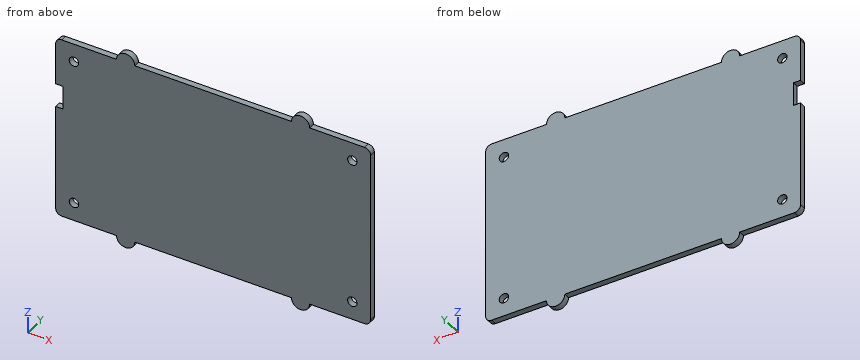
from build123d import *

# Parameters (mm, degrees)
SKETCH_1_R      = 1.55
EXTRUDE_1_DEPTH = 2


with BuildPart() as part:
    # 草图1 → 凸台-拉伸1 (new body)
    with BuildSketch(Plane(origin=(0, 0, 0), x_dir=(1, 0, 0), z_dir=(0, 1, 0))):
        with BuildLine():
            Line((97.46, -4), (97.46, 52.29))
            ThreePointArc((97.46, 52.29), (96.874213562, 53.704213562), (95.46, 54.29))
            Line((95.46, 54.29), (77.46, 54.29))
            ThreePointArc((77.46, 54.29), (74.46, 57.29), (71.46, 54.29))
            Line((71.46, 54.29), (20, 54.29))
            ThreePointArc((20, 54.29), (17, 57.29), (14, 54.29))
            Line((14, 54.29), (-4, 54.29))
            ThreePointArc((-4, 54.29), (-5.414213562, 53.704213562), (-6, 52.29))
            Line((-6, 52.29), (-6, 17.493898271))
            Line((-6, 17.493898271), (-3.6, 17.493898271))
            Line((-3.6, 17.493898271), (-3.6, 9.75))
            Line((-3.6, 9.75), (-6, 9.75))
            Line((-6, 9.75), (-6, -4))
            ThreePointArc((-6, -4), (-5.414213562, -5.414213562), (-4, -6))
            Line((-4, -6), (14, -6))
            ThreePointArc((14, -6), (17, -9), (20, -6))
            Line((20, -6), (71.46, -6))
            ThreePointArc((71.46, -6), (74.46, -9), (77.46, -6))
            Line((77.46, -6), (95.46, -6))
            ThreePointArc((95.46, -6), (96.874213562, -5.414213562), (97.46, -4))
        make_face()
        Circle(SKETCH_1_R, mode=Mode.SUBTRACT)
        with Locations((91.46, 0)):
            Circle(SKETCH_1_R, mode=Mode.SUBTRACT)
        with Locations((0, 48.29)):
            Circle(SKETCH_1_R, mode=Mode.SUBTRACT)
        with Locations((91.46, 48.29)):
            Circle(SKETCH_1_R, mode=Mode.SUBTRACT)
    extrude(amount=EXTRUDE_1_DEPTH)


solid = part.part
Geometry check sheet. Reference: the model listing, model coordinates, mm. Round coordinates to 2 decimals unless told otherwise and drop trailing zeros. Order: outer loops, then holes, each group sorted by start corner. A loop starts at its lowest first (then second) coordinate and runs counter-clockwise, first axis right, second up. Notation, with made-up numbers: M -12,-28 L 15,-28 A21 cw 15,-1 Z; hole C 66.25,42.5 d8. An arc over 180 degrees is marked long. Answer in a Markdown table with one row per item. Add a question column.
Item 1: Sectioned sample at B-B, the plane z = 0. Enter the section's corners in (x, y).
Item 2: Depth check by flat-ended pin: pin 1 Ø0.6 at (x, y) = (6, 1) entering from +Z; pin 2 Ø1 at (x, y) = (-4.5, 1) entering from -Z; pin 3 Ø3 at (x, z) = (91.46, -48.29) entering from -Y; pin 4 Ø1 at (y, z) = (1, -14.5) entering from -X. Enter the tip coordinate at first touch or a pass-through.
Item 3: Sectioned sample at C-C, the plane y = 0.9. Enter the section's corners in (x, z), plus the area to 3 significant figures.
Item 4: Material ranges on L1, parallel to X at y = 1.4, z = -48.29; L2, parallel to Z at x = 0, y = 0.45; L3, parallel to Z at x = 89, y = 0.9, recorded low to high. Write a range as [from, to].
Item 5: Sectioned sample at A-A, the plane x = 0. Enter the section's corners in (y, z), plus the area to 3 significant figures.
Item 6: Sectioned sample at D-D, the plane x = 82.5. Enter the section's corners in (y, z), plus the area to 3 significant figures.
Filled in:
| question | item | result |
|---|---|---|
| 1 | outline | M -6,0 L -1.55,0 L -1.55,2 L -6,2 Z; M 1.55,0 L 89.91,0 L 89.91,2 L 1.55,2 Z; M 93.01,0 L 97.46,0 L 97.46,2 L 93.01,2 Z |
| 2 | pin 1 | stops at z = 6 |
| 2 | pin 2 | stops at z = -54.29 |
| 2 | pin 3 | passes through |
| 2 | pin 4 | stops at x = -3.6 |
| 3 | outline | M -6,-52.29 A2 ccw -4,-54.29 L 14,-54.29 A3 ccw 20,-54.29 L 71.46,-54.29 A3 ccw 77.46,-54.29 L 95.46,-54.29 A2 ccw 97.46,-52.29 L 97.46,4 A2 ccw 95.46,6 L 77.46,6 A3 ccw 71.46,6 L 20,6 A3 ccw 14,6 L -4,6 A2 ccw -6,4 L -6,-9.75 L -3.6,-9.75 L -3.6,-17.49 L -6,-17.49 Z; hole C 0,-48.29 d3.1; hole C 0,0 d3.1; hole C 91.46,-48.29 d3.1; hole C 91.46,0 d3.1 |
| 3 | area | 6,240 mm² |
| 4 | L1 | x = [-6, -1.55], [1.55, 89.91], [93.01, 97.46] |
| 4 | L2 | z = [-54.29, -49.84], [-46.74, -1.55], [1.55, 6] |
| 4 | L3 | z = [-54.29, 6] |
| 5 | outline | M 0,-54.29 L 2,-54.29 L 2,-49.84 L 0,-49.84 Z; M 0,-46.74 L 2,-46.74 L 2,-1.55 L 0,-1.55 Z; M 0,1.55 L 2,1.55 L 2,6 L 0,6 Z |
| 5 | area | 108 mm² |
| 6 | outline | M 0,-54.29 L 2,-54.29 L 2,6 L 0,6 Z |
| 6 | area | 121 mm² |
